```python
from build123d import *

# Parameters (mm, degrees)
BOSS_EXTRUDE1_DEPTH = 2
SKETCH3_W           = 430
SKETCH3_H           = 2
BOSS_EXTRUDE2_DEPTH = 30
CUT_EXTRUDE1_DEPTH  = 50
SKETCH7_R           = 4
CUT_EXTRUDE2_DEPTH  = 445.998876403
SKETCH8_R           = 4
CUT_EXTRUDE3_DEPTH  = 445.998876403
BOSS_EXTRUDE4_REACH = 466.157
FILLET3_R           = 1


with BuildPart() as part:
    # Sketch2 → Boss-Extrude1 (new body)
    with BuildSketch(Plane.XY):
        Polygon((0, 0), (430, 0), (430, 25), (0, 110), align=None)
    extrude(amount=BOSS_EXTRUDE1_DEPTH)

    # Sketch3 → Boss-Extrude2 (add)
    with BuildSketch(Plane(origin=(0, 0, 0), x_dir=(-1, 0, 0), z_dir=(0, 0, -1))):
        with Locations((-215, 1)):
            Rectangle(SKETCH3_W, SKETCH3_H)
    extrude(amount=BOSS_EXTRUDE2_DEPTH)

    # Sketch4 → Cut-Extrude1 (cut)
    with BuildSketch(Plane(origin=(0, 2, 0), x_dir=(1, 0, 0), z_dir=(0, 1, 0))):
        with BuildLine():
            Line((40, 20), (120, 20))
            ThreePointArc((120, 20), (125, 15), (120, 10))
            Line((120, 10), (40, 10))
            ThreePointArc((40, 10), (35, 15), (40, 20))
        make_face()
        with BuildLine():
            Line((390, 20), (310, 20))
            ThreePointArc((310, 20), (305, 15), (310, 10))
            Line((310, 10), (390, 10))
            ThreePointArc((390, 10), (395, 15), (390, 20))
        make_face()
    extrude(amount=-CUT_EXTRUDE1_DEPTH, mode=Mode.SUBTRACT)

    # Sketch7 → Cut-Extrude2 (cut, through all)
    with BuildSketch(Plane.XY.offset(2)):
        with Locations((15, 50)):
            Circle(SKETCH7_R)
        with Locations((50, 15)):
            Circle(SKETCH7_R)
        with Locations((390, 15)):
            Circle(SKETCH7_R)
        with Locations((15, 90)):
            Circle(SKETCH7_R)
    extrude(amount=-CUT_EXTRUDE2_DEPTH, mode=Mode.SUBTRACT)

    # Sketch8 → Cut-Extrude3 (cut, through all)
    with BuildSketch(Plane.XY.offset(2)):
        with Locations((140, 10)):
            Circle(SKETCH8_R)
        with Locations((220, 10)):
            Circle(SKETCH8_R)
        with Locations((300, 10)):
            Circle(SKETCH8_R)
    extrude(amount=-CUT_EXTRUDE3_DEPTH, mode=Mode.SUBTRACT)

    # Boss-Extrude4: up to this plane
    boss_extrude4_end = Plane(origin=(430, 0, 2), z_dir=(-1, 0, 0))
    # Sketch12 → Boss-Extrude4 (add, up to the surface)
    with BuildSketch(Plane(origin=(-20.926480156, 4.136629798, 0), x_dir=(0, 0, -1), z_dir=(0.9810169593645325, -0.19392195708368665, 0)), mode=Mode.PRIVATE) as boss_extrude4_sk1:
        with BuildLine():
            Line((2.668468057, 109.913216573), (0, 107.91186553))
            Line((0, 107.91186553), (-2, 107.91186553))
            Line((-2, 107.91186553), (-2, 108.91186553))
            Line((-2, 108.91186553), (1.468468057, 111.513216573))
            ThreePointArc((1.468468057, 111.513216573), (2.868468057, 111.313216573), (2.668468057, 109.913216573))
        make_face()
    boss_extrude4_tool1 = split(extrude(boss_extrude4_sk1.sketch, amount=BOSS_EXTRUDE4_REACH, mode=Mode.PRIVATE), bisect_by=boss_extrude4_end, keep=Keep.BOTH, mode=Mode.PRIVATE)
    add(boss_extrude4_tool1.solids().sort_by_distance((0.341058, 111.725355, -0.613229))[0])

    # Fillet3
    fillet3_edges = [part.edges().sort_by_distance(p)[0] for p in [
        (215.096960979, 68.500183664, 2),
        (215, 67.5, 0),
    ]]
    fillet(fillet3_edges, radius=FILLET3_R)


solid = part.part
```
For this review, take the finished solid that the model builds, in its own axes (mm). A direction names the side the tool comes from. Round coordinates to 2 decimals unless told otherwise and drop trailing zeros.
Q1. Machinability: for faces 4 (the cylindrical face through (218.15, 67.85, 1.89)), 5 (the flat face through (164, 45, 0)), which of the approach directions +Z, -Z, +X, -X, +Y, -Y give a long, thin tool a straight path to every point of the face, cutting with its end or side? Answer none if there is none.
Findings below:
face 4: +Z, +X, +Y
face 5: -Z, -X
Q2. Insertion check: P1, Ø8, axis at x = 370.5, z = -22, coming from the +Y side; P2, Ø13, axis at x = 15, y = 90, coming from the -Z side; P3, Ø15, axis at x = 189, z = -9, coming from the +Y side. Each pin has a flat end and moves straight along its axis. Give the tip position at first contact, or say it passes through.
Findings below:
P1: stops at y = 2
P2: stops at z = 0
P3: stops at y = 77.16
Q3. Mouldability with a two-part tool opening along X and no side actions: class faces 1 (the flat face through (0, 38.4, 0.3)), 2 (the flat face through (218, 2, -15)), 3 (the cylindrical face through (216, 10, 1)) as pulls with the +X half, pulls with the -X half, needs draft (parallel to the pull), parting line crosses it, or undercut.
Findings below:
face 1: pulls with the -X half
face 2: needs draft
face 3: undercut
Q4. We need section A-A, the plane x = 50. State how many separate pieces and enclosed holes the cut face has, plus the area to 3 significant figures.
Findings below:
separate pieces: 3
enclosed holes: 0
area: 235 mm2
Q5. Wall thickness on line 1 (Y direction, x = 332, z = -21.5); line 2 (Y direction, x = 15, z = 1.2): over which ranges is each line inside the solid? List them lowest first.
Findings below:
line 1: y = 0 to 2
line 2: y = 0 to 46, 54 to 86, 94 to 108.67
